from build123d import *

# Parameters (mm, degrees)
BOSS_EXTRUDE1_DEPTH     = 1.27
CUT_EXTRUDE1_DEPTH      = 373.740805793
CUT_EXTRUDE1_DEPTH_BACK = 373.740805793
SKETCH2_R               = 2.54
CUT_EXTRUDE2_DEPTH      = 373.740805793
CUT_EXTRUDE2_DEPTH_BACK = 373.740805793
SKETCH3_R               = 2.54
FILLET2_R               = 2.54


with BuildPart() as part:
    # Sketch1 → Boss-Extrude1 (new, symmetric)
    with BuildSketch(Plane(origin=(0, 0, 0), x_dir=(1, 0, 0), z_dir=(0, 1, 0))):
        Polygon((-34.188416223, -6.711856618), (-2.438416223, -6.711856618), (-2.438416223, 367.938143382), (-59.588416223, 367.938143382), (-59.588416223, 101.238143382), (-34.188416223, 101.238143382), align=None)
    extrude(amount=BOSS_EXTRUDE1_DEPTH, both=True)

    # Sketch2 → Cut-Extrude1 (cut, two sides: drawn at the far end of the back side and taken through both)
    with BuildSketch(Plane(origin=(0, 1.27, 0), x_dir=(1, 0, 0), z_dir=(0, 1, 0)).offset(-CUT_EXTRUDE1_DEPTH_BACK)):
        with Locations(Location((-27.838416223, 18.688143382, 0), (0, 0, 270))):
            Circle(SKETCH2_R)
        with Locations(Location((-8.788416223, 18.688143382, 0), (0, 0, 270))):
            Circle(SKETCH2_R)
        with Locations(Location((-8.788416223, 28.340143382, 0), (0, 0, 270))):
            Circle(SKETCH2_R)
        with Locations(Location((-8.788416223, 37.992143382, 0), (0, 0, 270))):
            Circle(SKETCH2_R)
        with Locations(Location((-27.838416223, 28.340143382, 0), (0, 0, 270))):
            Circle(SKETCH2_R)
        with Locations(Location((-27.838416223, 37.992143382, 0), (0, 0, 270))):
            Circle(SKETCH2_R)
    extrude(amount=CUT_EXTRUDE1_DEPTH + CUT_EXTRUDE1_DEPTH_BACK, mode=Mode.SUBTRACT)

    # Sketch3 → Cut-Extrude2 (cut, two sides: drawn at the far end of the back side and taken through both)
    with BuildSketch(Plane(origin=(0, 1.27, 0), x_dir=(1, 0, 0), z_dir=(0, 1, 0)).offset(-CUT_EXTRUDE2_DEPTH_BACK)):
        with Locations(Location((-50.063416223, 126.638143382, 0), (0, 0, 270))):
            Circle(SKETCH3_R)
        with Locations(Location((-11.963416223, 126.638143382, 0), (0, 0, 270))):
            Circle(SKETCH3_R)
        with Locations(Location((-11.963416223, 152.038143382, 0), (0, 0, 270))):
            Circle(SKETCH3_R)
        with Locations(Location((-11.963416223, 177.438143382, 0), (0, 0, 270))):
            Circle(SKETCH3_R)
        with Locations(Location((-11.963416223, 202.838143382, 0), (0, 0, 270))):
            Circle(SKETCH3_R)
        with Locations(Location((-11.963416223, 228.238143382, 0), (0, 0, 270))):
            Circle(SKETCH3_R)
        with Locations(Location((-11.963416223, 253.638143382, 0), (0, 0, 270))):
            Circle(SKETCH3_R)
        with Locations(Location((-11.963416223, 279.038143382, 0), (0, 0, 270))):
            Circle(SKETCH3_R)
        with Locations(Location((-11.963416223, 304.438143382, 0), (0, 0, 270))):
            Circle(SKETCH3_R)
        with Locations(Location((-11.963416223, 329.838143382, 0), (0, 0, 270))):
            Circle(SKETCH3_R)
        with Locations(Location((-11.963416223, 355.238143382, 0), (0, 0, 270))):
            Circle(SKETCH3_R)
        with Locations(Location((-50.063416223, 152.038143382, 0), (0, 0, 270))):
            Circle(SKETCH3_R)
        with Locations(Location((-50.063416223, 177.438143382, 0), (0, 0, 270))):
            Circle(SKETCH3_R)
        with Locations(Location((-50.063416223, 202.838143382, 0), (0, 0, 270))):
            Circle(SKETCH3_R)
        with Locations(Location((-50.063416223, 228.238143382, 0), (0, 0, 270))):
            Circle(SKETCH3_R)
        with Locations(Location((-50.063416223, 253.638143382, 0), (0, 0, 270))):
            Circle(SKETCH3_R)
        with Locations(Location((-50.063416223, 279.038143382, 0), (0, 0, 270))):
            Circle(SKETCH3_R)
        with Locations(Location((-50.063416223, 304.438143382, 0), (0, 0, 270))):
            Circle(SKETCH3_R)
        with Locations(Location((-50.063416223, 329.838143382, 0), (0, 0, 270))):
            Circle(SKETCH3_R)
        with Locations(Location((-50.063416223, 355.238143382, 0), (0, 0, 270))):
            Circle(SKETCH3_R)
    extrude(amount=CUT_EXTRUDE2_DEPTH + CUT_EXTRUDE2_DEPTH_BACK, mode=Mode.SUBTRACT)

    # Fillet2
    fillet2_edges = [part.edges().sort_by_distance(p)[0] for p in [
        (-34.188416223, 0, -101.238143382),
        (-59.588416223, 0, -101.238143382),
        (-59.588416223, 0, -367.938143382),
        (-2.438416223, 0, -367.938143382),
        (-2.438416223, 0, 6.711856618),
        (-34.188416223, 0, 6.711856618),
    ]]
    fillet(fillet2_edges, radius=FILLET2_R)


solid = part.part
Verification items for the finished model (mm, model axes). Round coordinates to 2 decimals unless told otherwise and drop trailing zeros. Order: outer loops, then holes, each group sorted by start corner. A loop starts at its lowest first (then second) coordinate and runs counter-clockwise, first axis right, second up. Notation, with made-up numbers: (1, -15) -> (20, -15) arc R24 cw to (20, 23) -> close; hole circle Ø2 at (43.5, 67). An arc over 180 degrees is marked (long way). Put each result on its own line as item: value.
1) Section check B-B (y = -0.6). Give the number of separate pieces and of enclosed holes in the cut face, then the cut area to 3 significant figures.
Final values:
separate pieces: 1
enclosed holes: 26
area: 18,100 mm^2
2) Section check A-A (x = -43.5). Record the cut outline in (y, z), then the cut area to 3 significant figures.
Final values:
outline: (-1.27, -367.94) -> (1.27, -367.94) -> (1.27, -101.24) -> (-1.27, -101.24) -> close
area: 677 mm^2
3) Material ranges on line 1 (Z direction, x = -8.5, y = 0.9); line 2 (X direction, y = 0.5, z = -125); line 3 (Z direction, x = -4.5, y = 0.7), recorded low to high.
Final values:
line 1: z = -367.94 to -40.52, -35.47 to -30.86, -25.82 to -21.21, -16.16 to 6.71
line 2: x = -59.59 to -52, -48.12 to -13.9, -10.02 to -2.44
line 3: z = -367.89 to 6.67
